```python
from build123d import *

# Parameters (mm, degrees)
SKETCH_1_W          = 55.5
SKETCH_1_H          = 23.5
EXTRUDE_1_DEPTH     = 1.2
FILLET_1_R          = 2
SKETCH_2_W          = 53.7
SKETCH_2_H          = 22.3
EXTRUDE_2_DEPTH     = 0.6
SKETCH_3_W          = 13
SKETCH_3_H          = 14
SKETCH_3_W_2        = 13.5
SKETCH_3_W_3        = 14
SKETCH_3_H_2        = 13.05
CUT_EXTRUDE_1_DEPTH = 3
FILLET_2_R          = 1
SKETCH_4_W          = 15.5
SKETCH_4_H          = 3.997435945
CUT_EXTRUDE_2_DEPTH = 0.5
SKETCH_5_W          = 53.5
SKETCH_5_H          = 1.5
EXTRUDE_3_DEPTH     = 6.5
FILLET_3_R          = 1
SKETCH_6_W          = 1.5
SKETCH_6_H          = 4
EXTRUDE_4_DEPTH     = 3.75
CHAMFER_1_SIZE      = 2
FILLET_4_R          = 1.5


with BuildPart() as part:
    # 草图1 → 凸台-拉伸1 (new body)
    with BuildSketch(Plane(origin=(0, 0, 0), x_dir=(1, 0, 0), z_dir=(0, 1, 0))):
        Rectangle(SKETCH_1_W, SKETCH_1_H)
    extrude(amount=EXTRUDE_1_DEPTH)

    # 圆角1
    fillet_1_edges = [part.edges().sort_by_distance(p)[0] for p in [
        (27.75, 0.6, 11.75),
        (-27.75, 0.6, 11.75),
        (-27.75, 0.6, -11.75),
        (27.75, 0.6, -11.75),
    ]]
    fillet(fillet_1_edges, radius=FILLET_1_R)

    # 草图2 → 凸台-拉伸2 (add)
    with BuildSketch(Plane.XZ):
        Rectangle(SKETCH_2_W, SKETCH_2_H)
    extrude(amount=EXTRUDE_2_DEPTH)

    # 草图3 → 切除-拉伸1 (cut)
    with BuildSketch(Plane.XZ.offset(0.6)):
        with Locations((-19.05, 3.85)):
            Rectangle(SKETCH_3_W, SKETCH_3_H)
        with Locations((-1, 3.85)):
            Rectangle(SKETCH_3_W_2, SKETCH_3_H)
        with Locations((17.95, 2.516421356)):
            Rectangle(SKETCH_3_W_3, SKETCH_3_H_2)
    extrude(amount=-CUT_EXTRUDE_1_DEPTH, mode=Mode.SUBTRACT)

    # 圆角2
    fillet_2_edges = [part.edges().sort_by_distance(p)[0] for p in [
        (-25.55, 0.3, -3.15),
        (-25.55, 0.3, 10.85),
        (-12.55, 0.3, 10.85),
        (-12.55, 0.3, -3.15),
        (-7.75, 0.3, -3.15),
        (-7.75, 0.3, 10.85),
        (5.75, 0.3, 10.85),
        (5.75, 0.3, -3.15),
        (10.95, 0.3, -4.008578644),
        (10.95, 0.3, 9.041421356),
        (24.95, 0.3, 9.041421356),
        (24.95, 0.3, -4.008578644),
    ]]
    fillet(fillet_2_edges, radius=FILLET_2_R)

    # 草图4 → 切除-拉伸2 (cut)
    with BuildSketch(Plane(origin=(0, 1.2, 0), x_dir=(1, 0, 0), z_dir=(0, 1, 0))):
        with Locations((-20, -3.751282028)):
            Rectangle(SKETCH_4_W, SKETCH_4_H)
    extrude(amount=-CUT_EXTRUDE_2_DEPTH, mode=Mode.SUBTRACT)

    # 草图5 → 凸台-拉伸3 (add)
    with BuildSketch(Plane(origin=(0, 1.2, 0), x_dir=(1, 0, 0), z_dir=(0, 1, 0))):
        with Locations((0, 6.804632487)):
            Rectangle(SKETCH_5_W, SKETCH_5_H)
    extrude(amount=EXTRUDE_3_DEPTH)

    # 圆角3
    fillet_3_edges = [part.edges().sort_by_distance(p)[0] for p in [
        (26.75, 7.7, -6.804632487),
        (-26.75, 7.7, -6.804632487),
    ]]
    fillet(fillet_3_edges, radius=FILLET_3_R)

    # 草图6 → 凸台-拉伸4 (add)
    with BuildSketch(Plane(origin=(0, 1.2, 0), x_dir=(1, 0, 0), z_dir=(0, 1, 0))):
        with Locations((9, 4.054632487)):
            Rectangle(SKETCH_6_W, SKETCH_6_H)
        with Locations((-11, 4.054632487)):
            Rectangle(SKETCH_6_W, SKETCH_6_H)
    extrude(amount=EXTRUDE_4_DEPTH)

    # 倒角1
    chamfer_1_edges = [part.edges().sort_by_distance(p)[0] for p in [
        (9, 4.95, -2.054632487),
        (-11, 4.95, -2.054632487),
    ]]
    chamfer(chamfer_1_edges, length=CHAMFER_1_SIZE)

    # 圆角4
    fillet_4_edges = [part.edges().sort_by_distance(p)[0] for p in [
        (-26.85, -0.3, 11.15),
        (-26.85, -0.3, -11.15),
        (26.85, -0.3, -11.15),
        (26.85, -0.3, 11.15),
    ]]
    fillet(fillet_4_edges, radius=FILLET_4_R)


solid = part.part
```
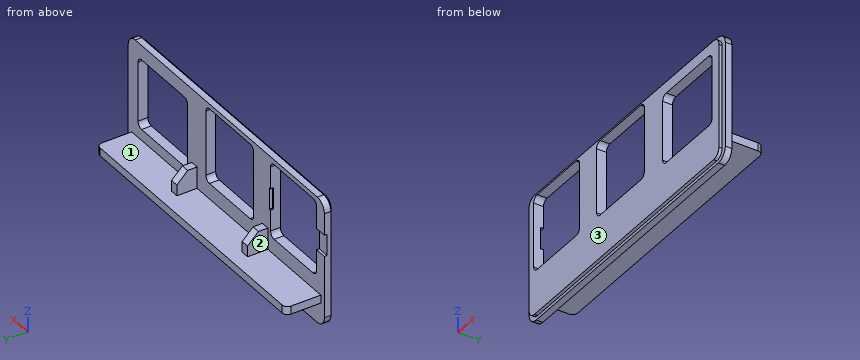
Here's how the part is built. I have some questions about the finished solid (model axes, mm). Face numbers are marked on the shaded views. Coordinates: 2 decimals unless noted, no trailing zeros. Order: outer loops, then holes, each group sorted by start corner. A loop starts at its lowest first (then second) coordinate and runs counter-clockwise, first axis right, second up. Notation, with made-up numbers: M 59.25,89 L 101.25,89 A31 ccw 101.25,127 Z; hole C 28,51.25 d7. An arc over 180 degrees is marked long. Answer as a JSON object with one key per item and string values. Group by question number.
(1) Suppose I cut it at B-B, the plane x = 13. Please give me the cut outline in (y, z), then the cut area to 3 significant figures.
(2) I need wall thicknesses on probe 1 along X at (y, z) = (1.5, -4.75); probe 2 along Z at (x, y) = (-25, 4); probe 3 along Y at (x, z) = (-23, -4.5). Which ranges of each line are inside material? Lowest first, please.
(3) For pin 1 (3 mm diameter, centred on x = 18.5, y = 4, fed in from +Z); pin 2 (1.1 mm diameter, centred on x = -26.5, z = 3, fed in from +Y); pin 3 (1.2 mm diameter, centred on y = 5, z = -7, fed in from -X), each with a flat end and sliding along its axis, tell me the tip position at first contact or that it passes through.
(4) If we mould it in two halves opening along X, with no side actions, what happens to the marked faces 1, 2 and 3? For each: released by +X, released by -X, zero draft, split by the parting line, or undercut.
(5) Suppose I cut it at C-C, the plane y = 1.75. Please give me the cut outline in (x, z).
(6) Suppose I cut it at D-D, the plane z = -7. Please give me the cut outline in (x, y), then the cut area to 3 significant figures.
(7) Suppose I cut it at A-A, the plane z = 2.25. Please give me the cut outline in (x, y), then the cut area to 3 significant figures.
Values found:
{
 "1": {"outline": "M -0.6,-11.15 L 0,-11.15 L 0,-11.75 L 1.2,-11.75 L 1.2,-7.55 L 7.7,-7.55 L 7.7,-6.05 L 1.2,-6.05 L 1.2,-4.01 L -0.6,-4.01 Z; M -0.6,9.04 L 1.2,9.04 L 1.2,11.75 L 0,11.75 L 0,11.15 L -0.6,11.15 Z", "area": "27.8 mm^2"},
 "2": {"probe 1": "x = -11.75 to -10.25, 8.25 to 9.75", "probe 2": "z = -7.55 to -6.05", "probe 3": "y = -0.6 to 1.2"},
 "3": {"pin 1": "stops at z = -6.05", "pin 2": "stops at y = 0.7", "pin 3": "stops at x = -26.75"},
 "4": {"face 1": "undercut", "face 2": "released by -X", "face 3": "zero draft"},
 "5": {"outline": "M -26.75,-7.55 L 26.75,-7.55 L 26.75,-6.05 L 9.75,-6.05 L 9.75,-2.05 L 8.25,-2.05 L 8.25,-6.05 L -10.25,-6.05 L -10.25,-2.05 L -11.75,-2.05 L -11.75,-6.05 L -26.75,-6.05 Z"},
 "6": {"outline": "M -27.75,0 L -26.85,0 L -26.85,-0.6 L 26.85,-0.6 L 26.85,0 L 27.75,0 L 27.75,1.2 L 26.75,1.2 L 26.75,6.7 A1 ccw 25.75,7.7 L -25.75,7.7 A1 ccw -26.75,6.7 L -26.75,1.2 L -27.75,1.2 Z", "area": "446 mm^2"},
 "7": {"outline": "M -27.75,0 L -26.85,0 L -26.85,-0.6 L -25.55,-0.6 L -25.55,0.7 L -27.75,0.7 Z; M -12.55,-0.6 L -7.75,-0.6 L -7.75,1.2 L -12.25,1.2 L -12.25,0.7 L -12.55,0.7 Z; M 5.75,-0.6 L 10.95,-0.6 L 10.95,1.2 L 5.75,1.2 Z; M 24.95,-0.6 L 26.85,-0.6 L 26.85,0 L 27.75,0 L 27.75,1.2 L 24.95,1.2 Z", "area": "24.7 mm^2"}
}
